from build123d import *

# Parameters (mm, degrees)
SKETCH1_R           = 2.25
BOSS_EXTRUDE1_DEPTH = 3.175
FILLET1_R           = 6.35
FILLET2_R           = 1


with BuildPart() as part:
    # Sketch1 → Boss-Extrude1 (new body)
    with BuildSketch(Plane.XY):
        Polygon((0, 0), (-76.2, 0), (-76.2, 34.380256121), (-50.8, 59.780256121), (-50.8, 76.2), (-25.4, 76.2), (-25.4, 59.780256121), (0, 34.380256121), align=None)
        with Locations((-44.45, 57.15)):
            Circle(SKETCH1_R, mode=Mode.SUBTRACT)
        with Locations((-69.85, 6.35)):
            Circle(SKETCH1_R, mode=Mode.SUBTRACT)
        with Locations((-6.35, 6.35)):
            Circle(SKETCH1_R, mode=Mode.SUBTRACT)
        with Locations((-31.75, 44.45)):
            Circle(SKETCH1_R, mode=Mode.SUBTRACT)
        with Locations((-44.45, 44.45)):
            Circle(SKETCH1_R, mode=Mode.SUBTRACT)
        with Locations((-57.15, 6.35)):
            Circle(SKETCH1_R, mode=Mode.SUBTRACT)
        with Locations((-57.15, 31.75)):
            Circle(SKETCH1_R, mode=Mode.SUBTRACT)
        with Locations((-69.85, 31.75)):
            Circle(SKETCH1_R, mode=Mode.SUBTRACT)
        with Locations((-19.05, 6.35)):
            Circle(SKETCH1_R, mode=Mode.SUBTRACT)
        with Locations((-19.05, 31.75)):
            Circle(SKETCH1_R, mode=Mode.SUBTRACT)
        with Locations((-6.35, 31.75)):
            Circle(SKETCH1_R, mode=Mode.SUBTRACT)
        with Locations((-44.45, 31.75)):
            Circle(SKETCH1_R, mode=Mode.SUBTRACT)
        with Locations((-31.75, 31.75)):
            Circle(SKETCH1_R, mode=Mode.SUBTRACT)
        with Locations((-44.45, 19.05)):
            Circle(SKETCH1_R, mode=Mode.SUBTRACT)
        with Locations((-31.75, 19.05)):
            Circle(SKETCH1_R, mode=Mode.SUBTRACT)
        with Locations((-44.45, 6.35)):
            Circle(SKETCH1_R, mode=Mode.SUBTRACT)
        with Locations((-31.75, 6.35)):
            Circle(SKETCH1_R, mode=Mode.SUBTRACT)
        with Locations((-31.75, 57.15)):
            Circle(SKETCH1_R, mode=Mode.SUBTRACT)
        with Locations((-31.75, 69.85)):
            Circle(SKETCH1_R, mode=Mode.SUBTRACT)
        with Locations((-44.45, 69.85)):
            Circle(SKETCH1_R, mode=Mode.SUBTRACT)
        Polygon((-63.5, 38.1), (-50.8, 50.8), (-50.8, 38.1), align=None, mode=Mode.SUBTRACT)
        Polygon((-25.4, 50.8), (-25.4, 38.1), (-12.7, 38.1), align=None, mode=Mode.SUBTRACT)
    extrude(amount=BOSS_EXTRUDE1_DEPTH)

    # Fillet1
    fillet1_edges = [part.edges().sort_by_distance(p)[0] for p in [
        (0, 0, 1.5875),
        (-76.2, 0, 1.5875),
        (-76.2, 34.380256121, 1.5875),
        (-50.8, 59.780256121, 1.5875),
        (-50.8, 76.2, 1.5875),
        (-25.4, 76.2, 1.5875),
        (-25.4, 59.780256121, 1.5875),
        (0, 34.380256121, 1.5875),
    ]]
    fillet(fillet1_edges, radius=FILLET1_R)

    # Fillet2
    fillet2_edges = [part.edges().sort_by_distance(p)[0] for p in [
        (-63.5, 38.1, 1.5875),
        (-50.8, 38.1, 1.5875),
        (-50.8, 50.8, 1.5875),
        (-12.7, 38.1, 1.5875),
        (-25.4, 50.8, 1.5875),
        (-25.4, 38.1, 1.5875),
    ]]
    fillet(fillet2_edges, radius=FILLET2_R)


solid = part.part
Work out the finished part from the listing and answer in its coordinate system (mm). A direction names the side the tool comes from. Coordinates: 2 decimals unless noted, no trailing zeros. Write each loop counter-clockwise with the first axis right and the second up, starting at its lowest first coordinate (ties: lowest second). Pieces come first, ordered by that corner, then holes. Notation, with made-up numbers: M 15.25,27 L 48.25,27 A23 ccw 48.25,46 Z; hole C 58,-7.75 d6. An arc over 180 degrees is marked long. Write item = value, one per line.
1. The part is cut by section B-B (x = -65.5). Determine the outline of the cut face in (y, z) (3 decimals).
Solution:
outline = M 0,0 L 45.08,0 L 45.08,3.175 L 0,3.175 Z
2. For faces 5 (the face through (-50.8, 44, 2)), 6 (the face through (-25.4, 66, 2)), 7 (the face through (-38, 0, 2)), determine the directions among +Z, -Z, +X, -X, +Y, -Y from which every point of the face is accessible in a straight line to the end or side of a thin tool.
Solution:
face_5 = +Z, -Z
face_6 = +Z, -Z, +X, +Y
face_7 = +Z, -Z, +X, -X, -Y
3. The part is cut by section A-A (z = 1.8). State how many separate pieces and enclosed holes the cut face has, then the cut area to 3 significant figures.
Solution:
separate_pieces = 1
enclosed_holes = 22
area = 3,820 mm2
4. Determine the mould class of faces 1 (the face through (-30.712, 17.054, 1.565)), 2 (the face through (-44.74, 33.98, 1.57)), 3 (the face through (-51.297, 59.948, 1.61)), 4 (the face through (-74.29, 1.81, 1.61)) for opening direction Y: released by +Y, released by -Y, zero draft, split by the parting line, or undercut.
Solution:
face_1 = undercut
face_2 = undercut
face_3 = released by +Y
face_4 = released by -Y
5. Flat-ended cylindrical pins translate along their axes: pin 1 (1.5 mm diameter, centred on y = 40, z = 2, fed in from -X); pin 2 (1 mm diameter, centred on x = -30.5, z = 1.5, fed in from +Y); pin 3 (1 mm diameter, centred on y = 42.5, z = 2, fed in from +X); pin 4 (3.5 mm diameter, centred on x = -19.05, y = 6.35, fed in from +Z). Find the tip coordinate at first contact, or state that the pin passes through.
Solution:
pin_1 = -71.33
pin_2 = 76.16
pin_3 = -7.62
pin_4 = through
6. Straight lines are drawn through the part: line 1 (X direction, y = 48, z = 0.9); line 2 (Y direction, x = -68.5, z = 2.15); line 3 (X direction, y = 20.5, z = 1.1). For each, find the intervals that lie inside material, in ascending order. Write a range as from..to.
Solution:
line_1 = -62.58..-53.6, -50.8..-25.4, -22.6..-13.62
line_2 = 0..4.55, 8.15..29.95, 33.55..42.08
line_3 = -76.2..-46.17, -42.73..-33.47, -30.03..0
